Design review of the part built by this model. Coordinates are the model's own, in mm. Face numbers are marked on the shaded views. A direction names the side the tool comes from. Give positions to 0.01 mm unless a question says otherwise; leave off trailing zeros. Loops run counter-clockwise (first coordinate to the right, second up) from the corner with the lowest first, then second, coordinate; pieces in that order, holes last. Notation, with made-up numbers: (59, 41.25) -> (95, 41.25) arc R22 ccw to (95, 54.25) -> close; hole circle Ø7 at (27.25, -23). An arc over 180 degrees is marked (long way). Answer as CSV lines item,"result".
from build123d import *

# Parameters (mm, degrees)
SKETCH_1_W      = 90
SKETCH_1_H      = 90
EXTRUDE_1_DEPTH = 168
FILLET_1_R      = 10
SKETCH_2_R      = 27.5
EXTRUDE_2_DEPTH = 10
SKETCH_3_R      = 30
EXTRUDE_3_DEPTH = 17


with BuildPart() as part:
    # 스케치1 → 보스-돌출1 (new body)
    with BuildSketch(Plane.XY):
        with Locations((45, -45)):
            Rectangle(SKETCH_1_W, SKETCH_1_H)
    extrude(amount=EXTRUDE_1_DEPTH)

    # 필렛1
    fillet_1_edges = [part.edges().sort_by_distance(p)[0] for p in [
        (90, -45, 168),
        (45, 0, 168),
        (0, -45, 168),
        (45, 0, 0),
        (90, -45, 0),
        (45, -90, 0),
        (0, -45, 0),
        (45, -90, 168),
        (0, 0, 84),
        (90, 0, 84),
        (90, -90, 84),
        (0, -90, 84),
    ]]
    fillet(fillet_1_edges, radius=FILLET_1_R)

    # 스케치2 → 보스-돌출2 (add)
    with BuildSketch(Plane.XY.offset(168)):
        with Locations((45, -45)):
            Circle(SKETCH_2_R)
    extrude(amount=EXTRUDE_2_DEPTH)

    # 스케치3 → 보스-돌출3 (add)
    with BuildSketch(Plane.XY.offset(178)):
        with Locations((45, -45)):
            Circle(SKETCH_3_R)
    extrude(amount=EXTRUDE_3_DEPTH)


solid = part.part
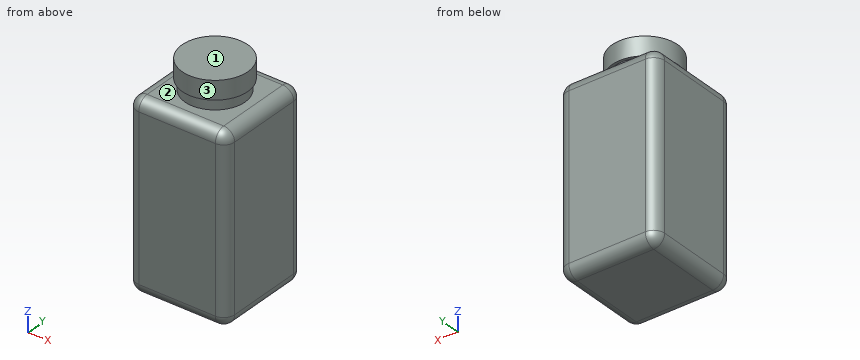
Q1. We need section D-D, the plane x = 84.5. State the section outline as (y, z) points, and give its area (3 significant figures).
Filled sheet:
outline,"(-88.93, 10) arc R8.93 ccw to (-80, 1.07) -> (-10, 1.07) arc R8.93 ccw to (-1.07, 10) -> (-1.07, 158) arc R8.93 ccw to (-10, 166.93) -> (-80, 166.93) arc R8.93 ccw to (-88.93, 158) -> close"
area,"14,500 mm^2"
Q2. We need section B-B, the plane x = 45. State the section outline as (y, z) points, and give its area (3 significant figures).
Filled sheet:
outline,"(-90, 10) arc R10 ccw to (-80, 0) -> (-10, 0) arc R10 ccw to (0, 10) -> (0, 158) arc R10 ccw to (-10, 168) -> (-17.5, 168) -> (-17.5, 178) -> (-15, 178) -> (-15, 195) -> (-75, 195) -> (-75, 178) -> (-72.5, 178) -> (-72.5, 168) -> (-80, 168) arc R10 ccw to (-90, 158) -> close"
area,"16,600 mm^2"
Q3. Clearance check with a flat-ended pin moving along its axis: pin 1 Ø6 at (x, z) = (47.5, 159.5) entering from -Y. State where the tip first meets the part, or that it passes through.
Filled sheet:
pin 1,"stops at y = -90"
Q4. For the marked faces 1, 2 and 3, list the 3-axis set-ups (+Z, -Z, +X, -X, +Y, -Y) from which the entire face can be reached by the end or side of a thin tool; tool diameter is ignored.
Filled sheet:
face 1,"+Z, +X, -X, +Y, -Y"
face 2,"none"
face 3,"+Z"
Q5. We need section C-C, the plane z = 162. State the section outline as (x, y) points.
Filled sheet:
outline,"(0.83, -80) arc R9.17 ccw to (10, -89.17) -> (80, -89.17) arc R9.17 ccw to (89.17, -80) -> (89.17, -10) arc R9.17 ccw to (80, -0.83) -> (10, -0.83) arc R9.17 ccw to (0.83, -10) -> close"
Q6. To check wall thickness, follow probe 1 along Z at (x, y) = (75.5, -24.5); probe 2 along Z at (x, y) = (7, -82.5); probe 3 along Y at (x, z) = (37.5, 163.5). State the ranges of each line that lie inside material, in increasing order. Write a range as from..to.
Filled sheet:
probe 1,"z = 0..168"
probe 2,"z = 0.79..167.21"
probe 3,"y = -88.35..-1.65"
Q7. We need section A-A, the plane y = -45. State the section outline as (x, z) points, and give its area (3 significant figures).
Filled sheet:
outline,"(0, 10) arc R10 ccw to (10, 0) -> (80, 0) arc R10 ccw to (90, 10) -> (90, 158) arc R10 ccw to (80, 168) -> (72.5, 168) -> (72.5, 178) -> (75, 178) -> (75, 195) -> (15, 195) -> (15, 178) -> (17.5, 178) -> (17.5, 168) -> (10, 168) arc R10 ccw to (0, 158) -> close"
area,"16,600 mm^2"
